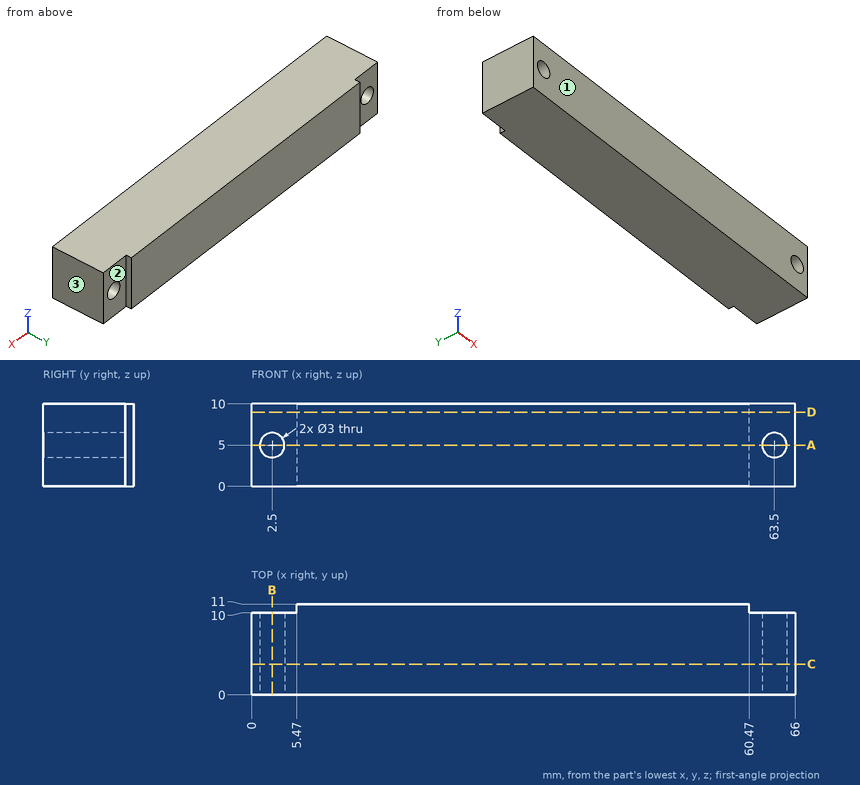
The figure shows three views and two pictorial views of one solid part (mm, origin at its lowest corner). Answer the questions. Give positions to 0.01 mm unless a question says otherwise; leave off trailing zeros. Loops run counter-clockwise (first coordinate to the right, second up) from the corner with the lowest first, then second, coordinate; pieces in that order, holes last. Notation, with made-up numbers: (56, 48.5) - (101, 48.5) arc R16 ccw to (101, 62.5) - close; hole circle Ø9 at (41, 72.5). An arc over 180 degrees is marked (long way). Answer in a Markdown table with one row per item.
(1) Section B-B (x = 2.5) is taken. Give the vertices of the cut face in (y, z), and give its area (3 significant figures).
Results list:
| item | result |
|---|---|
| outline | (0, 0) - (10, 0) - (10, 3.5) - (0, 3.5) - close; (0, 6.5) - (10, 6.5) - (10, 10) - (0, 10) - close |
| area | 70.0 mm² |
(2) Flat-ended cylindrical pins translate along their axes: pin 1 Ø4 at (x, z) = (54.5, 8) entering from -Y; pin 2 Ø1.8 at (x, z) = (2.5, 5) entering from +Y; pin 3 Ø0.8 at (y, z) = (10.5, 6) entering from +X; pin 4 Ø0.5 at (y, z) = (10.5, 6) entering from -X. Find the tip coordinate at first contact, or state that the pin passes through.
Results list:
| item | result |
|---|---|
| pin 1 | stops at y = 0 |
| pin 2 | passes through |
| pin 3 | stops at x = 60.47 |
| pin 4 | stops at x = 5.47 |
(3) Section D-D (z = 9) is taken. Give the vertices of the cut face in (x, y), and give its area (3 significant figures).
Results list:
| item | result |
|---|---|
| outline | (0, 0) - (66, 0) - (66, 10) - (60.47, 10) - (60.47, 11) - (5.47, 11) - (5.47, 10) - (0, 10) - close |
| area | 715 mm² |
(4) Consider L1, parallel to X at y = 5.75, z = 5; L2, parallel to Z at x = 2.5, y = 6; L3, parallel to X at y = 6.75, z = 6.25. Determine where each line is inside the solid, lowest interval first. Write a range as [from, to].
Results list:
| item | result |
|---|---|
| L1 | x = [0, 1], [4, 62], [65, 66] |
| L2 | z = [0, 3.5], [6.5, 10] |
| L3 | x = [0, 1.67], [3.33, 62.67], [64.33, 66] |
(5) Section A-A (z = 5) is taken. Give the vertices of the cut face in (x, y), and give its area (3 significant figures).
Results list:
| item | result |
|---|---|
| outline | (0, 0) - (1, 0) - (1, 10) - (0, 10) - close; (4, 0) - (62, 0) - (62, 10) - (60.47, 10) - (60.47, 11) - (5.47, 11) - (5.47, 10) - (4, 10) - close; (65, 0) - (66, 0) - (66, 10) - (65, 10) - close |
| area | 655 mm² |
(6) For a pull along Y with two mould halves and no side action, classify the marked faces 1, 2 and 3 as pulls with the +Y half, pulls with the -Y half, needs draft (parallel to the pull), parting line crosses it, or undercut.
Results list:
| item | result |
|---|---|
| face 1 | pulls with the -Y half |
| face 2 | pulls with the +Y half |
| face 3 | needs draft |
(7) Section C-C (y = 3.75) is taken. Give the vertices of the cut face in (x, z), and give its area (3 significant figures).
Results list:
| item | result |
|---|---|
| outline | (0, 0) - (66, 0) - (66, 10) - (0, 10) - close; hole circle Ø3 at (2.5, 5); hole circle Ø3 at (63.5, 5) |
| area | 646 mm² |
